Geometry: see drawing. Coordinates: mm, zero at the bounding-box minimum. A direction names the side the tool comes from. Give positions to 0.01 mm unless a question says otherwise; leave off trailing zeros. Write each loop counter-clockwise with the first axis right and the second up, starting at its lowest first coordinate (ties: lowest second). Pieces come first, ordered by that corner, then holes. Notation, with made-up numbers: (73.5, 10.25) -> (123.5, 10.25) arc R29 ccw to (123.5, 35.25) -> close; hole circle Ø10 at (52.5, 87.5). An arc over 180 degrees is marked (long way). Answer as a JSON object with one key per item and string values. Group by question number.
Item 1: Section query D-D on x = 38.5. Return the cut outline in (y, z).
Item 2: Section query A-A on x = 124. Return the cut outline in (y, z).
Item 3: Section query C-C on x = 14. Return the cut outline in (y, z), plus the area to 3 significant figures.
Item 4: Pull-direction query (X, two-part tool) for the marked faces 3 and 4; classes: pulls with the +X half, pulls with the -X half, needs draft (parallel to the pull), parting line crosses it, or undercut.
Item 5: Section query B-B on y = 2.5. Return the cut outline in (x, z) (1 decimal), plus the area to 3 significant figures.
Item 6: Ray query, probe 1 along Z at (x, y) = (14, 4.5); probe 2 along Z at (x, y) = (124, 10.5); probe 3 along X at (y, z) = (13.25, 22.5) (1 decimal). Return the intervals inside material, ascending. Write a range as from..to.
Item 7: Access query for the marked faces 1 and 2. Directions: +Z, -Z, +X, -X, +Y, -Y. A direction counts if a zero-diameter tool reaches every point of the face in a straight line with its end or side. Return the directions, or none.
Item 8: First-contact query: pin 1 Ø5 at (x, z) = (92, 40) entering from -Y; pin 2 Ø18 at (x, z) = (14, 29) entering from -Y; pin 3 Ø8 at (x, y) = (43.5, 3.5) entering from +Z; pin 4 Ø1 at (y, z) = (10, 35.5) entering from -X. Flat tips, straight axial feed; report the tip coordinate or a pass-through.
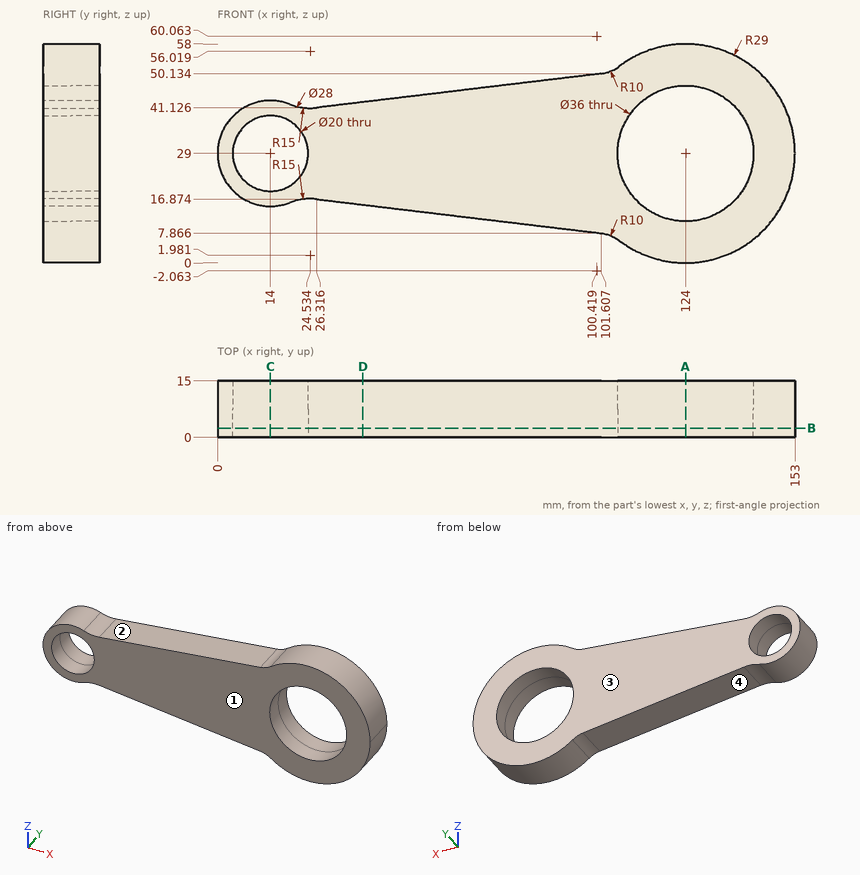
Worked answers:
{
 "1": {"outline": "(0, 15.42) -> (15, 15.42) -> (15, 42.58) -> (0, 42.58) -> close"},
 "2": {"outline": "(0, 0) -> (15, 0) -> (15, 11) -> (0, 11) -> close; (0, 47) -> (15, 47) -> (15, 58) -> (0, 58) -> close"},
 "3": {"outline": "(0, 15) -> (15, 15) -> (15, 19) -> (0, 19) -> close; (0, 39) -> (15, 39) -> (15, 43) -> (0, 43) -> close", "area": "120 mm^2"},
 "4": {"face 3": "needs draft", "face 4": "undercut"},
 "5": {"outline": "(19.1, 16) arc R15 cw to (26.3, 16.9) -> (101.6, 7.9) arc R10 cw to (106.5, 5.9) arc R29 ccw (long way) to (106.5, 52.1) arc R10 cw to (101.6, 50.1) -> (26.3, 41.1) arc R15 cw to (19.1, 42) arc R14 ccw (long way) to start; hole circle Ø20 at (14, 29); hole circle Ø36 at (124, 29)", "area": "4,280 mm^2"},
 "6": {"probe 1": "15..19, 39..43", "probe 2": "0..11, 47..58", "probe 3": "1.6..6.4, 21.6..107.2, 140.8..152.3"},
 "7": {"face 1": "+Z, -Z, +X, -X, -Y", "face 2": "+Z, +Y, -Y"},
 "8": {"pin 1": "y = 0", "pin 2": "through", "pin 3": "z = 43.66", "pin 4": "x = 1.35"}
}
